The listing builds one solid part. Answer for the finished solid, in the listing's coordinates (mm). Face numbers are marked on the shaded views. A direction names the side the tool comes from. Coordinates: 2 decimals unless noted, no trailing zeros. Loops run counter-clockwise (first coordinate to the right, second up) from the corner with the lowest first, then second, coordinate; pieces in that order, holes last. Notation, with made-up numbers: M 80,-16.75 L 89,-16.75 A32 cw 89,16.25 Z; hole C 38.25,16.25 d7. An arc over 180 degrees is marked long. Answer as a JSON object with one key per item and string values. Group by question number.
1. Determine the mould class of the marked faces 1, 2, 3 and 4 for opening direction Z: released by +Z, released by -Z, zero draft, split by the parting line, or undercut.
2. A cutting plane is placed at D-D on z = 4. Give the vertices of the cut face in (x, y), and give its area (3 significant figures).
3. Straight lines are drawn through the part: L1, parallel to Z at x = 9.25, y = -2; L2, parallel to Z at x = 12, y = 43.5; L3, parallel to Y at x = 9.5, z = 18.75. For each, find the intervals that lie inside material, in ascending order.
4. A cutting plane is placed at A-A on x = 6.25. Give the vertices of the cut face in (y, z), and give its area (3 significant figures).
5. For the marked faces 5 and 6, determine the directions among +Z, -Z, +X, -X, +Y, -Y from which every point of the face is accessible in a straight line to the end or side of a thin tool.
6. Given pin 1 (1 mm diameter, centred on y = 21, z = 20, fed in from -X), flat-ended and moving along its own axis, determine where the tip first touches the part or whether it passes through.
7. A cutting plane is placed at C-C on y = -2. Give the vertices of the cut face in (x, z).
8. A cutting plane is placed at B-B on z = 16.5. Give the vertices of the cut face in (x, y), and give its area (3 significant figures).
from build123d import *

# Parameters (mm, degrees)
SKETCH1_W           = 29
SKETCH1_H           = 47
BOSS_EXTRUDE1_DEPTH = 26
SHELL1_T            = -3
SKETCH2_W           = 10
SKETCH2_H           = 8.23076923
CUT_EXTRUDE1_DEPTH  = 26
SKETCH3_W           = 29
SKETCH3_H           = 26
BOSS_EXTRUDE2_DEPTH = 20
SKETCH4_R           = 2.5
CUT_EXTRUDE2_DEPTH  = 62.040969848


with BuildPart() as part:
    # Sketch1 → Boss-Extrude1 (new body)
    with BuildSketch(Plane.XY):
        with Locations((14.5, 23.5)):
            Rectangle(SKETCH1_W, SKETCH1_H)
    extrude(amount=BOSS_EXTRUDE1_DEPTH)

    # Shell1
    shell1_openings = [part.faces().sort_by_distance(p)[0] for p in [
        (0, 23.5, 13),
    ]]
    offset(amount=SHELL1_T, openings=shell1_openings, kind=Kind.INTERSECTION)

    # Sketch2 → Cut-Extrude1 (cut)
    with BuildSketch(Plane.ZY):
        with Locations((13, 44)):
            Rectangle(SKETCH2_W, SKETCH2_H)
    extrude(amount=-CUT_EXTRUDE1_DEPTH, mode=Mode.SUBTRACT)

    # Sketch3 → Boss-Extrude2 (add)
    with BuildSketch(Plane.XZ):
        with Locations((14.5, 13)):
            Rectangle(SKETCH3_W, SKETCH3_H)
    extrude(amount=BOSS_EXTRUDE2_DEPTH)

    # Sketch4 → Cut-Extrude2 (cut, through all)
    with BuildSketch(Plane.ZY):
        with Locations(Location((8, -2, 0), (0, 0, 270))):
            Circle(SKETCH4_R)
        with Locations(Location((18, -2, 0), (0, 0, 270))):
            Circle(SKETCH4_R)
    extrude(amount=-CUT_EXTRUDE2_DEPTH, mode=Mode.SUBTRACT)


solid = part.part
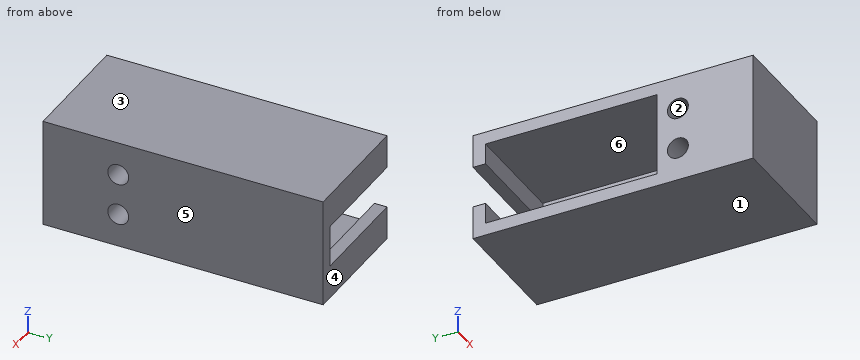
From the geometry:
{
 "1": {"face 1": "released by -Z", "face 2": "undercut", "face 3": "released by +Z", "face 4": "zero draft"},
 "2": {"outline": "M 0,-20 L 29,-20 L 29,47 L 0,47 L 0,44 L 26,44 L 26,3 L 0,3 Z", "area": "877 mm²"},
 "3": {"L1": "z = 0 to 5.5, 10.5 to 15.5, 20.5 to 26", "L2": "z = 0 to 3, 23 to 26", "L3": "y = -20 to -4.38, 0.38 to 3, 44 to 47"},
 "4": {"outline": "M -20,0 L 47,0 L 47,8 L 44,8 L 44,3 L 3,3 L 3,23 L 44,23 L 44,18 L 47,18 L 47,26 L -20,26 Z; hole C -2,8 d5; hole C -2,18 d5", "area": "853 mm²"},
 "5": {"face 5": "+Z, -Z, +X, +Y, -Y", "face 6": "-X"},
 "6": {"pin 1": "stops at x = 26"},
 "7": {"outline": "M 0,0 L 29,0 L 29,5.5 L 0,5.5 Z; M 0,10.5 L 29,10.5 L 29,15.5 L 0,15.5 Z; M 0,20.5 L 29,20.5 L 29,26 L 0,26 Z"},
 "8": {"outline": "M 0,-20 L 29,-20 L 29,-4 L 0,-4 Z; M 0,0 L 29,0 L 29,47 L 26,47 L 26,3 L 0,3 Z", "area": "683 mm²"}
}
